Could you check a few things on this model? Use its own coordinates, in mm. A direction names the side the tool comes from. Coordinates: 2 decimals unless noted, no trailing zeros. Order: outer loops, then holes, each group sorted by start corner. A loop starts at its lowest first (then second) coordinate and runs counter-clockwise, first axis right, second up. Notation, with made-up numbers: (84, 83) - (117, 83) arc R28 cw to (117, 120) - close; hole circle Ø6 at (43.5, -22.75). An arc over 180 degrees is marked (long way). One line per item, written item: value.
from build123d import *

# Parameters (mm, degrees)
SKETCH1_W           = 25.4
SKETCH1_H           = 25.4
SKETCH1_W_2         = 19.05
SKETCH1_H_2         = 19.05
BOSS_EXTRUDE1_DEPTH = 914.4
CUT_EXTRUDE1_REACH  = 27.4
SKETCH4_R           = 1.7145
CUT_EXTRUDE3_DEPTH  = 26.4
SKETCH6_R           = 1.5875
CUT_EXTRUDE5_DEPTH  = 26.4


with BuildPart() as part:
    # Sketch1 → Boss-Extrude1 (new body)
    with BuildSketch(Plane(origin=(0, 0, 0), x_dir=(1, 0, 0), z_dir=(0, 1, 0))):
        Rectangle(SKETCH1_W, SKETCH1_H)
        Rectangle(SKETCH1_W_2, SKETCH1_H_2, mode=Mode.SUBTRACT)
    extrude(amount=BOSS_EXTRUDE1_DEPTH)

    # Sketch2 → Cut-Extrude1 (cut, up to next)
    with BuildSketch(Plane(origin=(0, 0, 12.7), x_dir=(-1, 0, 0), z_dir=(0, 0, -1)), mode=Mode.PRIVATE) as cut_extrude1_sk1:
        with BuildLine():
            Line((-2.38125, 879.475), (-2.38125, 904.875))
            ThreePointArc((-2.38125, 904.875), (0, 907.25625), (2.38125, 904.875))
            Line((2.38125, 904.875), (2.38125, 879.475))
            ThreePointArc((2.38125, 879.475), (0, 877.09375), (-2.38125, 879.475))
        make_face()
    cut_extrude1_tool1 = extrude(cut_extrude1_sk1.sketch, amount=CUT_EXTRUDE1_REACH, mode=Mode.PRIVATE) & part.part
    add(cut_extrude1_tool1.solids().sort_by_distance((0, 892.175, 12.7))[0], mode=Mode.SUBTRACT)

    # Sketch4 → Cut-Extrude3 (cut, through all)
    with BuildSketch(Plane.ZY.offset(12.7)):
        with Locations((-6.35, 561.975)):
            Circle(SKETCH4_R)
        with Locations((6.35, 587.375)):
            Circle(SKETCH4_R)
        with Locations((-6.35, 612.775)):
            Circle(SKETCH4_R)
        with Locations((6.35, 638.175)):
            Circle(SKETCH4_R)
        with Locations((-6.35, 663.575)):
            Circle(SKETCH4_R)
        with Locations((6.35, 688.975)):
            Circle(SKETCH4_R)
        with Locations((-6.35, 714.375)):
            Circle(SKETCH4_R)
        with Locations((6.35, 739.775)):
            Circle(SKETCH4_R)
        with Locations((-6.35, 765.175)):
            Circle(SKETCH4_R)
        with Locations((6.35, 790.575)):
            Circle(SKETCH4_R)
        with Locations((-6.35, 815.975)):
            Circle(SKETCH4_R)
    extrude(amount=-CUT_EXTRUDE3_DEPTH, mode=Mode.SUBTRACT)

    # Sketch6 → Cut-Extrude5 (cut, through all)
    with BuildSketch(Plane.XY.offset(12.7)):
        with Locations((0, 19.05)):
            Circle(SKETCH6_R)
        with Locations((0, 38.1)):
            Circle(SKETCH6_R)
        with Locations((0, 57.15)):
            Circle(SKETCH6_R)
        with Locations((0, 76.2)):
            Circle(SKETCH6_R)
        with Locations((0, 95.25)):
            Circle(SKETCH6_R)
        with Locations((0, 114.3)):
            Circle(SKETCH6_R)
        with Locations((0, 133.35)):
            Circle(SKETCH6_R)
        with Locations((0, 152.4)):
            Circle(SKETCH6_R)
        with Locations((0, 171.45)):
            Circle(SKETCH6_R)
        with Locations((0, 190.5)):
            Circle(SKETCH6_R)
        with Locations((0, 209.55)):
            Circle(SKETCH6_R)
        with Locations((0, 228.6)):
            Circle(SKETCH6_R)
        with Locations((0, 247.65)):
            Circle(SKETCH6_R)
        with Locations((0, 266.7)):
            Circle(SKETCH6_R)
        with Locations((0, 285.75)):
            Circle(SKETCH6_R)
    extrude(amount=-CUT_EXTRUDE5_DEPTH, mode=Mode.SUBTRACT)


solid = part.part
Item 1: I'm going to push a flat-ended pin straight in: pin 1 Ø1.5 at (x, z) = (-7, 0.5) entering from -Y. Where does the tip first touch, or does it pass through?
Conclusion:
pin 1: through
Item 2: I want a section at B-B on z = 0.5. Please give me the cut outline in (x, y) (3 decimals).
Conclusion:
outline: (-12.7, 0) - (-9.525, 0) - (-9.525, 914.4) - (-12.7, 914.4) - close; (9.525, 0) - (12.7, 0) - (12.7, 914.4) - (9.525, 914.4) - close
Item 3: If I drill on probe 1 along X at (y, z) = (798, 6.5) (3 decimals); probe 2 along X at (y, z) = (133.35, 11.15), over which ranges is the centre line in solid material (lowest first)?
Conclusion:
probe 1: -12.7 to -9.525, 9.525 to 12.7
probe 2: -12.7 to -1.59, 1.59 to 12.7
Item 4: Thinking about a two-plate mould opening in X: for faces 3 (the face through (0, 451, 12.7)), 4 (the face through (-9.525, 451, 0)), 5 (the face through (9.525, 451, 0)), 6 (the face through (12.7, 451, 0)), which applies, pulls with the +X half, pulls with the -X half, needs draft (parallel to the pull), parting line crosses it, or undercut?
Conclusion:
face 3: needs draft
face 4: undercut
face 5: undercut
face 6: pulls with the +X half
Item 5: I want a section at A-A on y = 468. Please give me the cut outline in (x, z) (3 decimals).
Conclusion:
outline: (-12.7, -12.7) - (12.7, -12.7) - (12.7, 12.7) - (-12.7, 12.7) - close; hole (-9.525, -9.525) - (9.525, -9.525) - (9.525, 9.525) - (-9.525, 9.525) - close
Item 6: For faces 1 (the face through (0, 451, 9.525)), 2 (the face through (0, 451, -12.7)), which set-ups out of +Z, -Z, +X, -X, +Y, -Y let a thin tool reach every point of the face, with its end or its side?
Conclusion:
face 1: +Y, -Y
face 2: -Z, +X, -X, +Y, -Y
